Autodesk Inventor part; units mm, degrees
ref_plane "YZ Plane" through (0, 0, 0) normal (1, 0, 0) x (0, 1, 0)
ref_plane "XZ Plane" through (0, 0, 0) normal (0, 1, 0) x (-1, 0, 0)
ref_plane "XY Plane" through (0, 0, 0) normal (0, 0, 1) x (1, 0, 0)
sketch "スケッチ1" plane through (0, 0, 0) normal (0, 0, 1) x (1, 0, 0)
  circle A0 centre (0, 0) radius 3
  circle A1 centre (0, 0) radius 1.25
  dimension "d0" = 6
  dimension "d1" = 2.5
extrude "押し出し1" add sketch "スケッチ1" along normal blind 20
chamfer "面取り1" distance 0.3 angle 45 4 edges at (-3, 0, 20) (-1.25, 0, 20) (-3, 0, 0) (-1.25, 0, 0)
thread "ねじ1"
properties part number "p9ALshaft" material "アルミニウム 2014-T4"
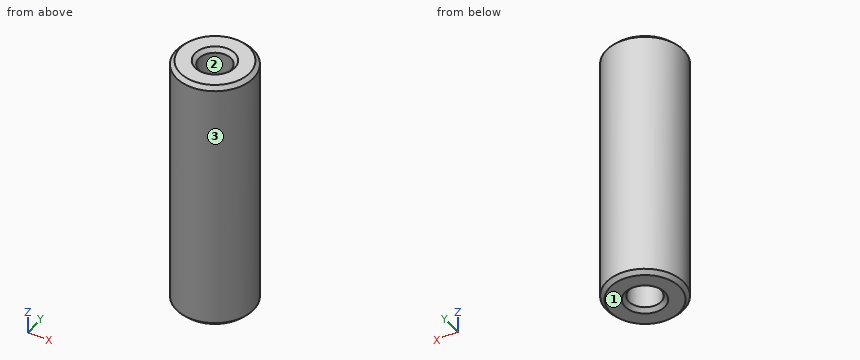
Can you work these out from the model? Positions are in its coordinate system, mm. Face numbers are marked on the shaded views. Give positions to 0.01 mm unless a question says otherwise; leave off trailing zeros. Write each loop counter-clockwise with the first axis right and the second up, starting at its lowest first coordinate (ties: lowest second). Pieces come first, ordered by that corner, then holes. Notation, with made-up numbers: (20.5, 9.25) -> (69.5, 9.25) arc R30 cw to (69.5, 48.25) -> close; hole circle Ø1 at (39.25, 62). An arc over 180 degrees is marked (long way). One line per item, written item: value.
Q1. Please list where these lines run through material, in increasing order: line 1 (Y direction, x = 0, z = 9.75); line 2 (X direction, y = 0.8, z = 6); line 3 (X direction, y = 0.15, z = 16). Write a range as [from, to].
Results found:
line 1: y = [-3, -1.25], [1.25, 3]
line 2: x = [-2.89, -0.96], [0.96, 2.89]
line 3: x = [-3, -1.24], [1.24, 3]
Q2. Imagine slicing it at A-A on x = 0. Please give me the cut outline in (y, z).
Results found:
outline: (-3, 0.3) -> (-2.7, 0) -> (-1.55, 0) -> (-1.25, 0.3) -> (-1.25, 19.7) -> (-1.55, 20) -> (-2.7, 20) -> (-3, 19.7) -> close; (1.25, 0.3) -> (1.55, 0) -> (2.7, 0) -> (3, 0.3) -> (3, 19.7) -> (2.7, 20) -> (1.55, 20) -> (1.25, 19.7) -> close
Q3. Imagine slicing it at C-C on z = 5.5. Please give me the cut outline in (x, y), and give its area (3 significant figures).
Results found:
outline: circle Ø6 at (0, 0); hole circle Ø2.5 at (0, 0)
area: 23.4 mm^2
Q4. For P1, Ø2, axis at y = -0.5, z = 11.5, coming from the -X side; P2, Ø1, axis at x = 1, z = 9, coming from the +Y side, each with a flat end and sliding along its axis, tell me the tip position at first contact or that it passes through.
Results found:
P1: stops at x = -3
P2: stops at y = 2.96
Q5. We'd pull the mould along Y, two halves only. Please class the marked faces 1, 2 and 3: +Y half, -Y half, draft (parallel to the pull), parting line (faces both ways), or undercut.
Results found:
face 1: draft
face 2: undercut
face 3: parting line
